The model under review builds one solid part; all positions refer to its coordinate system, in mm. A direction names the side the tool comes from. Give positions to 0.01 mm unless a question says otherwise; leave off trailing zeros. Loops run counter-clockwise (first coordinate to the right, second up) from the corner with the lowest first, then second, coordinate; pieces in that order, holes last. Notation, with made-up numbers: M 25.5,50 L 36.5,50 A30 cw 36.5,73 Z; hole C -7,28.5 d9. An arc over 180 degrees is marked long. Return JSON: item names as keys, results as strings.
```python
from build123d import *

# Parameters (mm, degrees)
SKETCH_1_W          = 84
SKETCH_1_H          = 42
EXTRUDE_1_DEPTH     = 3
SKETCH_2_W          = 4
SKETCH_2_H          = 42
EXTRUDE_2_DEPTH     = 19
SKETCH_3_W          = 84
SKETCH_3_H          = 42
EXTRUDE_3_DEPTH     = 3
SKETCH_5_W          = 76
SKETCH_5_H          = 3
EXTRUDE_4_DEPTH     = 42
CUT_EXTRUDE_1_REACH = 55.198
SKETCH_4_R          = 14.5
SKETCH_4_R_2        = 2
SKETCH_6_R          = 13.5
CUT_EXTRUDE_2_DEPTH = 3
SKETCH_7_R          = 13
CUT_EXTRUDE_3_DEPTH = 3
CUT_EXTRUDE_4_DEPTH = 54.197744313
SKETCH_9_R          = 1.5
CUT_EXTRUDE_5_DEPTH = 3
CUT_EXTRUDE_START   = -19
CUT_EXTRUDE_6_DEPTH = 19
FILLET_1_R          = 1.5


with BuildPart() as part:
    # 草图1 → 凸台-拉伸1 (new body)
    with BuildSketch(Plane(origin=(0, 0, 0), x_dir=(1, 0, 0), z_dir=(0, 1, 0))):
        Rectangle(SKETCH_1_W, SKETCH_1_H)
    extrude(amount=EXTRUDE_1_DEPTH)

    # 草图2 → 凸台-拉伸2 (add)
    with BuildSketch(Plane(origin=(0, 3, 0), x_dir=(1, 0, 0), z_dir=(0, 1, 0))):
        with Locations((-40, 0)):
            Rectangle(SKETCH_2_W, SKETCH_2_H)
        with Locations((40, 0)):
            Rectangle(SKETCH_2_W, SKETCH_2_H)
    extrude(amount=EXTRUDE_2_DEPTH)

    # 草图3 → 凸台-拉伸3 (add)
    with BuildSketch(Plane(origin=(0, 22, 0), x_dir=(1, 0, 0), z_dir=(0, 1, 0))):
        Rectangle(SKETCH_3_W, SKETCH_3_H)
    extrude(amount=EXTRUDE_3_DEPTH)

    # 草图5 → 凸台-拉伸4 (add)
    with BuildSketch(Plane.XY.offset(21)):
        with Locations((0, 17.5)):
            Rectangle(SKETCH_5_W, SKETCH_5_H)
    extrude(amount=-EXTRUDE_4_DEPTH)

    # 草图4 → 切除-拉伸1 (cut, up to next)
    with BuildSketch(Plane(origin=(0, 25, 0), x_dir=(1, 0, 0), z_dir=(0, 1, 0)), mode=Mode.PRIVATE) as cut_extrude_1_sk1:
        with Locations(Location((0, 0, 0), (0, 0, 270))):
            Circle(SKETCH_4_R)
    cut_extrude_1_tool1 = extrude(cut_extrude_1_sk1.sketch, amount=-CUT_EXTRUDE_1_REACH, mode=Mode.PRIVATE) & part.part
    # 草图4 → 切除-拉伸1 (cut, up to next)
    with BuildSketch(Plane(origin=(0, 25, 0), x_dir=(1, 0, 0), z_dir=(0, 1, 0)), mode=Mode.PRIVATE) as cut_extrude_1_sk2:
        with Locations(Location((12.374368671, 12.374368671, 0), (0, 0, 270))):
            Circle(SKETCH_4_R_2)
    cut_extrude_1_tool2 = extrude(cut_extrude_1_sk2.sketch, amount=-CUT_EXTRUDE_1_REACH, mode=Mode.PRIVATE) & part.part
    # 草图4 → 切除-拉伸1 (cut, up to next)
    with BuildSketch(Plane(origin=(0, 25, 0), x_dir=(1, 0, 0), z_dir=(0, 1, 0)), mode=Mode.PRIVATE) as cut_extrude_1_sk3:
        with Locations(Location((12.374368671, -12.374368671, 0), (0, 0, 270))):
            Circle(SKETCH_4_R_2)
    cut_extrude_1_tool3 = extrude(cut_extrude_1_sk3.sketch, amount=-CUT_EXTRUDE_1_REACH, mode=Mode.PRIVATE) & part.part
    # 草图4 → 切除-拉伸1 (cut, up to next)
    with BuildSketch(Plane(origin=(0, 25, 0), x_dir=(1, 0, 0), z_dir=(0, 1, 0)), mode=Mode.PRIVATE) as cut_extrude_1_sk4:
        with Locations(Location((-12.374368671, -12.374368671, 0), (0, 0, 270))):
            Circle(SKETCH_4_R_2)
    cut_extrude_1_tool4 = extrude(cut_extrude_1_sk4.sketch, amount=-CUT_EXTRUDE_1_REACH, mode=Mode.PRIVATE) & part.part
    # 草图4 → 切除-拉伸1 (cut, up to next)
    with BuildSketch(Plane(origin=(0, 25, 0), x_dir=(1, 0, 0), z_dir=(0, 1, 0)), mode=Mode.PRIVATE) as cut_extrude_1_sk5:
        with Locations(Location((-12.374368671, 12.374368671, 0), (0, 0, 270))):
            Circle(SKETCH_4_R_2)
    cut_extrude_1_tool5 = extrude(cut_extrude_1_sk5.sketch, amount=-CUT_EXTRUDE_1_REACH, mode=Mode.PRIVATE) & part.part
    add(cut_extrude_1_tool1.solids().sort_by_distance((0, 25, 0))[0], mode=Mode.SUBTRACT)
    add(cut_extrude_1_tool2.solids().sort_by_distance((12.374369, 25, -12.374369))[0], mode=Mode.SUBTRACT)
    add(cut_extrude_1_tool3.solids().sort_by_distance((12.374369, 25, 12.374369))[0], mode=Mode.SUBTRACT)
    add(cut_extrude_1_tool4.solids().sort_by_distance((-12.374369, 25, 12.374369))[0], mode=Mode.SUBTRACT)
    add(cut_extrude_1_tool5.solids().sort_by_distance((-12.374369, 25, -12.374369))[0], mode=Mode.SUBTRACT)

    # 草图6 → 切除-拉伸2 (cut)
    with BuildSketch(Plane(origin=(0, 19, 0), x_dir=(1, 0, 0), z_dir=(0, 1, 0))):
        with Locations(Location((0, 0, 0), (0, 0, 270))):
            Circle(SKETCH_6_R)
    extrude(amount=-CUT_EXTRUDE_2_DEPTH, mode=Mode.SUBTRACT)

    # 草图7 → 切除-拉伸3 (cut)
    with BuildSketch(Plane.XZ):
        with Locations(Location((0, 0, 0), (0, 0, 270))):
            Circle(SKETCH_7_R)
    extrude(amount=-CUT_EXTRUDE_3_DEPTH, mode=Mode.SUBTRACT)

    # 草图8 → 切除-拉伸4 (cut, through all)
    with BuildSketch(Plane(origin=(0, 25, 0), x_dir=(1, 0, 0), z_dir=(0, 1, 0))):
        with BuildLine():
            Line((42, -13), (38, -13))
            ThreePointArc((38, -13), (25, 0), (38, 13))
            Line((38, 13), (42, 13))
            Line((42, 13), (42, -13))
        make_face()
        with BuildLine():
            Line((-42, 13), (-38, 13))
            ThreePointArc((-38, 13), (-25, 0), (-38, -13))
            Line((-38, -13), (-42, -13))
            Line((-42, -13), (-42, 13))
        make_face()
    extrude(amount=-CUT_EXTRUDE_4_DEPTH, mode=Mode.SUBTRACT)

    # 草图9 → 切除-拉伸5 (cut)
    with BuildSketch(Plane.XZ):
        with Locations(Location((33.412744657, 17.02464374, 0), (0, 0, 270))):
            Circle(SKETCH_9_R)
        with Locations(Location((-33.412744657, 17.02464374, 0), (0, 0, 90))):
            Circle(SKETCH_9_R)
        with Locations(Location((33.412744657, -17.02464374, 0), (0, 0, 90))):
            Circle(SKETCH_9_R)
        with Locations(Location((-33.412744657, -17.02464374, 0), (0, 0, 270))):
            Circle(SKETCH_9_R)
    extrude(amount=-CUT_EXTRUDE_5_DEPTH, mode=Mode.SUBTRACT)

    # 草图10 → 切除-拉伸6 (cut)
    with BuildSketch(Plane.XZ.offset(CUT_EXTRUDE_START)):
        with BuildLine():
            Line((7.25, 12.557368355), (11.25, 19.485571585))
            ThreePointArc((11.25, 19.485571585), (15.909902577, 15.909902577), (19.485571585, 11.25))
            Line((19.485571585, 11.25), (12.557368355, 7.25))
            ThreePointArc((12.557368355, 7.25), (10.253048327, 10.253048327), (7.25, 12.557368355))
        make_face()
        with BuildLine():
            Line((12.557368355, -7.25), (19.485571585, -11.25))
            ThreePointArc((19.485571585, -11.25), (15.909902577, -15.909902577), (11.25, -19.485571585))
            Line((11.25, -19.485571585), (7.25, -12.557368355))
            ThreePointArc((7.25, -12.557368355), (10.253048327, -10.253048327), (12.557368355, -7.25))
        make_face()
        with BuildLine():
            Line((-7.25, -12.557368355), (-11.25, -19.485571585))
            ThreePointArc((-11.25, -19.485571585), (-15.909902577, -15.909902577), (-19.485571585, -11.25))
            Line((-19.485571585, -11.25), (-12.557368355, -7.25))
            ThreePointArc((-12.557368355, -7.25), (-10.253048327, -10.253048327), (-7.25, -12.557368355))
        make_face()
        with BuildLine():
            Line((-12.557368355, 7.25), (-19.485571585, 11.25))
            ThreePointArc((-19.485571585, 11.25), (-15.909902577, 15.909902577), (-11.25, 19.485571585))
            Line((-11.25, 19.485571585), (-7.25, 12.557368355))
            ThreePointArc((-7.25, 12.557368355), (-10.253048327, 10.253048327), (-12.557368355, 7.25))
        make_face()
    extrude(amount=CUT_EXTRUDE_6_DEPTH, mode=Mode.SUBTRACT)

    # 圆角1
    fillet_1_edges = [part.edges().sort_by_distance(p)[0] for p in [
        (-11.25, 1.5, 19.485571585),
        (-19.485571585, 1.5, 11.25),
        (-12.557368355, 1.5, 7.25),
        (-7.25, 1.5, 12.557368355),
        (-11.25, 17.5, 19.485571585),
        (-19.485571585, 17.5, 11.25),
        (-12.557368355, 17.5, 7.25),
        (-7.25, 17.5, 12.557368355),
        (-19.485571585, 1.5, -11.25),
        (-11.25, 1.5, -19.485571585),
        (-7.25, 1.5, -12.557368355),
        (-12.557368355, 1.5, -7.25),
        (-19.485571585, 17.5, -11.25),
        (-11.25, 17.5, -19.485571585),
        (-7.25, 17.5, -12.557368355),
        (-12.557368355, 17.5, -7.25),
        (11.25, 1.5, -19.485571585),
        (19.485571585, 1.5, -11.25),
        (12.557368355, 1.5, -7.25),
        (7.25, 1.5, -12.557368355),
        (11.25, 17.5, -19.485571585),
        (19.485571585, 17.5, -11.25),
        (12.557368355, 17.5, -7.25),
        (7.25, 17.5, -12.557368355),
        (19.485571585, 1.5, 11.25),
        (11.25, 1.5, 19.485571585),
        (7.25, 1.5, 12.557368355),
        (12.557368355, 1.5, 7.25),
        (19.485571585, 17.5, 11.25),
        (11.25, 17.5, 19.485571585),
        (7.25, 17.5, 12.557368355),
        (12.557368355, 17.5, 7.25),
    ]]
    fillet(fillet_1_edges, radius=FILLET_1_R)


solid = part.part
```
1) Consider section D-D on x = -17. Write out the cut boundary in (y, z), then the cut area to 3 significant figures.
From the geometry:
{"outline": "M 0,-21 L 3,-21 L 3,-14.74 L 0,-14.74 Z; M 0,-9.81 L 3,-9.81 L 3,9.81 L 0,9.81 Z; M 0,14.74 L 3,14.74 L 3,21 L 0,21 Z; M 16,-21 L 19,-21 L 19,-14.74 L 16,-14.74 Z; M 16,-9.81 L 19,-9.81 L 19,9.81 L 16,9.81 Z; M 16,14.74 L 19,14.74 L 19,21 L 16,21 Z; M 22,-21 L 25,-21 L 25,21 L 22,21 Z", "area": "319 mm²"}
2) Insertion check: pin 1 (12 mm diameter, centred on y = 3.5, z = -4.5, fed in from +X); pin 2 (6 mm diameter, centred on y = 3, z = 4.5, fed in from -X); pin 3 (3 mm diameter, centred on x = -13, z = 14, fed in from -Y). Each pin has a flat end and moves straight along its axis. Give the tip position at first contact, or say it passes through.
From the geometry:
{"pin 1": "x = 30.31", "pin 2": "x = -27.38", "pin 3": "y = 22"}
3) Consider section C-C on z = 0. Write out the cut boundary in (x, y), then the cut area to 3 significant figures.
From the geometry:
{"outline": "M -25,0 L -13,0 L -13,3 L -25,3 Z; M -25,16 L -13.5,16 L -13.5,19 L -25,19 Z; M -25,22 L -14.5,22 L -14.5,25 L -25,25 Z; M 13,0 L 25,0 L 25,3 L 13,3 Z; M 13.5,16 L 25,16 L 25,19 L 13.5,19 Z; M 14.5,22 L 25,22 L 25,25 L 14.5,25 Z", "area": "204 mm²"}
4) Tool access review of faces 4 (the face through (-38, 20, -17)), 5 (the face through (-40, 13, -13)), 6 (the face through (10.6, 23.5, 13.3)), 7 (the face through (-15.87, 17.52, -15.95)): name each direction out of +Z, -Z, +X, -X, +Y, -Y from which nothing blocks a thin tool from reaching the whole face with its end or side.
From the geometry:
{"face 4": "+Z, -Z", "face 5": "-X, +Y, -Y", "face 6": "+Y, -Y", "face 7": "-Y"}
5) Wall thickness on L1, parallel to Y at x = 17.5, z = -9.5; L2, parallel to X at y = 19.5, z = 18; L3, parallel to X at y = 23.15, z = 0: over which ranges is each line inside the solid? List them lowest first. Write a range as from..to.
From the geometry:
{"L1": "0..3, 16..19, 22..25", "L2": "-42..-38, 38..42", "L3": "-25..-14.5, 14.5..25"}
6) Consider section A-A on y = 8. Write out the cut boundary in (x, z).
From the geometry:
{"outline": "M -42,-21 L -38,-21 L -38,-13 L -42,-13 Z; M -42,13 L -38,13 L -38,21 L -42,21 Z; M 38,-21 L 42,-21 L 42,-13 L 38,-13 Z; M 38,13 L 42,13 L 42,21 L 38,21 Z"}
7) Consider section B-B on x = 0. Write out the cut boundary in (y, z).
From the geometry:
{"outline": "M 0,-21 L 3,-21 L 3,-13 L 0,-13 Z; M 0,13 L 3,13 L 3,21 L 0,21 Z; M 16,-21 L 19,-21 L 19,-13.5 L 16,-13.5 Z; M 16,13.5 L 19,13.5 L 19,21 L 16,21 Z; M 22,-21 L 25,-21 L 25,-14.5 L 22,-14.5 Z; M 22,14.5 L 25,14.5 L 25,21 L 22,21 Z"}
8) The part is to be moulded in two halves that separate along Z. For faces 1 (the face through (-3, 17, 21)), 2 (the face through (-25, 18, 0)), 3 (the face through (-1, 19, 14)), say which applies: released by +Z, released by -Z, zero draft, split by the parting line, or undercut.
From the geometry:
{"face 1": "released by +Z", "face 2": "undercut", "face 3": "zero draft"}
